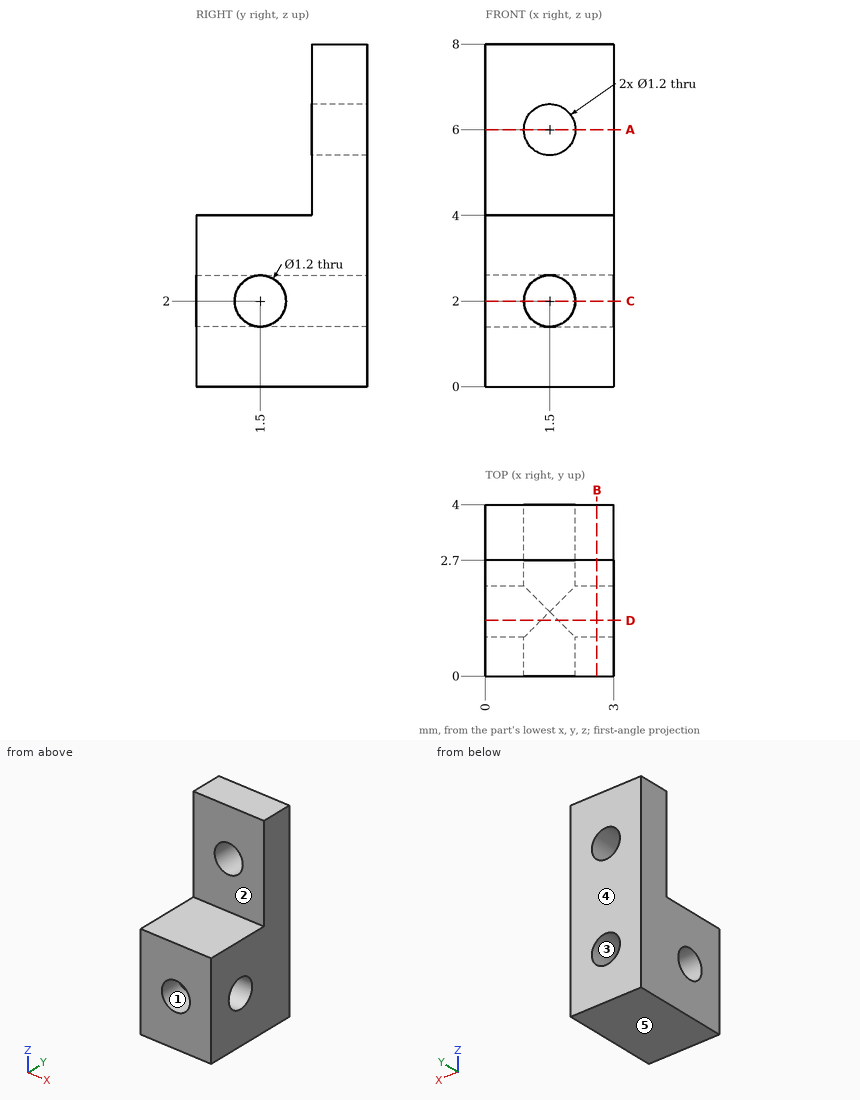
Answer from the drawing. Dimensions are ordinates in mm from the lowest x, y and z of the part. A direction names the side the tool comes from. Give positions to 0.01 mm unless a question says otherwise; leave off trailing zeros. Order: outer loops, then holes, each group sorted by start corner. A loop starts at its lowest first (then second) coordinate and runs counter-clockwise, first axis right, second up. Notation, with made-up numbers: (-23.75, 19.25) -> (24.25, 19.25) arc R20 ccw to (24.25, 40.25) -> close; hole circle Ø4 at (6, -11.75). An arc over 180 degrees is marked (long way). Answer as a JSON object with one key per item and string values. Group by question number.
1. Section B-B on x = 2.6 is taken. Determine the outline of the cut face in (y, z).
2. Section D-D on y = 1.3 is taken. Determine the outline of the cut face in (x, z), plus the area to 3 significant figures.
3. Section A-A on z = 6 is taken. Determine the outline of the cut face in (x, y), plus the area to 3 significant figures.
4. A tool of negligible diameter and unlimited length cuts with its end or side. For the marked faces 1 and 2, from which of +Z, -Z, +X, -X, +Y, -Y can it reach the whole face along a straight path? Write none if from no direction.
5. Consider line 1 along Z through (x, y) = (1.5, 3.35); line 2 along Z through (x, y) = (0.65, 1.5); line 3 along X through (y, z) = (2.8, 2). Determine where each line is inside the solid, lowest interval first. Write a range as [from, to].
6. Section C-C on z = 2 is taken. Determine the outline of the cut face in (x, y), plus the area to 3 significant figures.
7. The mould has two halves that part along Z. Classify the marked faces 3, 4 and 5: released by +Z, released by -Z, zero draft, split by the parting line, or undercut.
Result sheet:
{
 "1": {"outline": "(0, 0) -> (4, 0) -> (4, 8) -> (2.7, 8) -> (2.7, 4) -> (0, 4) -> close; hole circle Ø1.2 at (1.5, 2)"},
 "2": {"outline": "(0, 0) -> (3, 0) -> (3, 1.43) -> (1.7, 1.43) arc R0.6 cw to (1.3, 1.43) -> (0, 1.43) -> close; (0, 2.57) -> (1.3, 2.57) arc R0.6 cw to (1.7, 2.57) -> (3, 2.57) -> (3, 4) -> (0, 4) -> close", "area": "8.59 mm^2"},
 "3": {"outline": "(0, 2.7) -> (0.9, 2.7) -> (0.9, 4) -> (0, 4) -> close; (2.1, 2.7) -> (3, 2.7) -> (3, 4) -> (2.1, 4) -> close", "area": "2.34 mm^2"},
 "4": {"face 1": "+Y, -Y", "face 2": "+Z, +X, -X, -Y"},
 "5": {"line 1": "z = [0, 1.4], [2.6, 5.4], [6.6, 8]", "line 2": "z = [0, 1.4], [2.6, 4]", "line 3": "x = [0, 0.9], [2.1, 3]"},
 "6": {"outline": "(0, 0) -> (0.9, 0) -> (0.9, 0.9) -> (0, 0.9) -> close; (0, 2.1) -> (0.9, 2.1) -> (0.9, 4) -> (0, 4) -> close; (2.1, 0) -> (3, 0) -> (3, 0.9) -> (2.1, 0.9) -> close; (2.1, 2.1) -> (3, 2.1) -> (3, 4) -> (2.1, 4) -> close", "area": "5.04 mm^2"},
 "7": {"face 3": "undercut", "face 4": "zero draft", "face 5": "released by -Z"}
}
